```python
from build123d import *

# Parameters (mm, degrees)
BOSS_EXTRUDE1_DEPTH   = 46.39999966
SKETCH2_R             = 1.35
CUT_EXTRUDE1_DEPTH    = 57.705554564
CUT_EXTRUDE2_DEPTH    = 57.705554564
CUT_EXTRUDE3_DEPTH    = 77.912417193
MOVE_FACE1_BY         = 0.5
MOVE_FACE1_2_BY       = 0.5
CUT_EXTRUDE5_DEPTH    = 0.5
CUT_EXTRUDE6_DEPTH    = 0.5
MOVE_START            = 2.95
MOVE_FACE2_OUTLINE_W  = 4.2
MOVE_FACE2_OUTLINE_H  = 47.39999966
MOVE_FACE2_OUTLINE_R  = 1.35
MOVE_FACE2_DEPTH      = 2
MOVE_FACE3_BY         = 2
MOVE_FACE4_BY         = 0.1
MOVE_FACE4_2_BY       = 0.1
MOVE_FACE4_3_BY       = 0.1
MOVE_FACE4_4_BY       = 0.1
SKETCH14_W            = 31.645569848
SKETCH14_H            = 25
BOSS_EXTRUDE4_DEPTH   = 4
SKETCH15_R            = 2.1
CUT_EXTRUDE9_DEPTH    = 59.746648569
SKETCH16_R            = 3.6
CUT_EXTRUDE10_DEPTH   = 4.2
MOVE_FACE5_BY         = 4
MOVE_FACE6_BY         = 1
FILLET1_R             = 1
DELETEFACE1_START     = -5
DELETEFACE1_OUTLINE_R = 3.6
DELETEFACE1_DEPTH     = 6
DELETEFACE2_START     = -5
DELETEFACE2_OUTLINE_R = 1.35
DELETEFACE2_DEPTH     = 7.95
MOVE_FACE7_BY         = 4


# Read off the part's stored shape, not the designer's step: Move Face2, DeleteFace1, DeleteFace2
with BuildPart() as part:
    # Sketch1 → Boss-Extrude1 (new body)
    with BuildSketch(Plane.XY):
        Polygon((0, 0), (30, 0), (30, 12.7499), (22.3001, 12.7499), (22.3001, 9.7499), (26, 6.05), (26, 4.95), (22.3, 4.95), (22.3, 1), (0, 1), align=None)
    extrude(amount=-BOSS_EXTRUDE1_DEPTH)

    # Mirror1: part across plane


with BuildPart() as part_1:
    add(part.part)
    add(part.part.mirror(Plane(origin=(0, 1, -46.39999966), x_dir=(0, 0, 1), z_dir=(-1, 0, 0))))

    # Sketch2 → Cut-Extrude1 (cut, through all)
    with BuildSketch(Plane(origin=(0, 12.7499, 0), x_dir=(1, 0, 0), z_dir=(0, 1, 0))):
        with Locations(Location((-24.549999831, 1.999999999, 0), (0, 0, 270))):
            Circle(SKETCH2_R)
        with Locations(Location((-24.549999831, 44.399999661, 0), (0, 0, 270))):
            Circle(SKETCH2_R)
        with Locations(Location((24.549999831, 1.999999999, 0), (0, 0, 270))):
            Circle(SKETCH2_R)
        with Locations(Location((24.549999831, 44.399999661, 0), (0, 0, 270))):
            Circle(SKETCH2_R)
    extrude(amount=-CUT_EXTRUDE1_DEPTH, mode=Mode.SUBTRACT)

    # Sketch3 → Cut-Extrude2 (cut, through all)
    with BuildSketch(Plane.XY):
        Polygon((26.3, 12.7499), (30, 9.0499), (30, 12.7499), align=None)
        Polygon((-30, 12.7499), (-30, 9.0499), (-26.3, 12.7499), align=None)
    extrude(amount=-CUT_EXTRUDE2_DEPTH, mode=Mode.SUBTRACT)

    # Sketch4 → Cut-Extrude3 (cut, through all)
    with BuildSketch(Plane(origin=(30, 0, 0), x_dir=(0, 0, -1), z_dir=(1, 0, 0))):
        Polygon((9.19999983, 12.7499), (37.19999983, 12.7499), (30.416191902, 1), (15.983807758, 1), align=None)
    extrude(amount=-CUT_EXTRUDE3_DEPTH, mode=Mode.SUBTRACT)

    # Move Face1: a face moved outward by 0.5
    extrude(part_1.faces().sort_by_distance((-24, 3.187475, -46.39999966))[0], amount=MOVE_FACE1_BY, dir=(0, 0, -1))

    # Move Face1 2: a face moved outward by 0.5
    extrude(part_1.faces().sort_by_distance((-24, 3.187475, 0))[0], amount=MOVE_FACE1_2_BY, dir=(0, 0, 1))

    # Sketch6 → Cut-Extrude5 (cut)
    with BuildSketch(Plane(origin=(-26, 0, 0), x_dir=(0, 0, -1), z_dir=(1, 0, 0))):
        Polygon((13.703274195, 4.95), (13.068188899, 6.05), (-0.5, 6.05), (-0.5, 4.95), align=None)
        Polygon((33.331810761, 6.05), (32.696725465, 4.95), (46.89999966, 4.95), (46.89999966, 6.05), align=None)
    extrude(amount=-CUT_EXTRUDE5_DEPTH, mode=Mode.SUBTRACT)

    # Sketch7 → Cut-Extrude6 (cut)
    with BuildSketch(Plane.ZY.offset(-26)):
        Polygon((-13.068188899, 6.05), (-13.703274195, 4.95), (0.5, 4.95), (0.5, 6.05), align=None)
        Polygon((-32.696725465, 4.95), (-33.331810761, 6.05), (-46.89999966, 6.05), (-46.89999966, 4.95), align=None)
    extrude(amount=-CUT_EXTRUDE6_DEPTH, mode=Mode.SUBTRACT)

    # Move Face2 outline → Move Face2 (cut)
    # profile 1 of 2: a face of its own
    with BuildSketch(Plane(origin=(0, 0, 0), x_dir=(1, 0, 0), z_dir=(0, 1, 0)).offset(MOVE_START)):
        with Locations((-24.4, 23.19999983)):
            Rectangle(MOVE_FACE2_OUTLINE_W, MOVE_FACE2_OUTLINE_H)
        with Locations((-24.549999831, 1.999999999)):
            Circle(MOVE_FACE2_OUTLINE_R, mode=Mode.SUBTRACT)
        with Locations((-24.549999831, 44.399999661)):
            Circle(MOVE_FACE2_OUTLINE_R, mode=Mode.SUBTRACT)
    # profile 2 of 2: a face of its own
    with BuildSketch(Plane(origin=(0, 0, 0), x_dir=(1, 0, 0), z_dir=(0, 1, 0)).offset(MOVE_START)):
        with Locations((24.4, 23.19999983)):
            Rectangle(MOVE_FACE2_OUTLINE_W, MOVE_FACE2_OUTLINE_H)
        with Locations((24.549999831, 1.999999999)):
            Circle(MOVE_FACE2_OUTLINE_R, mode=Mode.SUBTRACT)
        with Locations((24.549999831, 44.399999661)):
            Circle(MOVE_FACE2_OUTLINE_R, mode=Mode.SUBTRACT)
    extrude(amount=MOVE_FACE2_DEPTH, mode=Mode.SUBTRACT)

    # Move Face3: a face moved outward by 2.0
    extrude(part_1.faces().sort_by_distance((0, 0, -23.19999983))[0], amount=MOVE_FACE3_BY, dir=(0, -1, 0))

    # Move Face4: a face moved inward by 0.1
    extrude(part_1.faces().sort_by_distance((-26.5, 4.468031617, -6.740769385))[0], amount=MOVE_FACE4_BY, dir=(-1, 0, 0), mode=Mode.SUBTRACT)

    # Move Face4 2: a face moved inward by 0.1
    extrude(part_1.faces().sort_by_distance((-26.5, 4.468031617, -39.659230275))[0], amount=MOVE_FACE4_2_BY, dir=(-1, 0, 0), mode=Mode.SUBTRACT)

    # Move Face4 3: a face moved inward by 0.1
    extrude(part_1.faces().sort_by_distance((26.5, 4.468031617, -6.740769385))[0], amount=MOVE_FACE4_3_BY, dir=(1, 0, 0), mode=Mode.SUBTRACT)

    # Move Face4 4: a face moved inward by 0.1
    extrude(part_1.faces().sort_by_distance((26.5, 4.468031617, -39.659230275))[0], amount=MOVE_FACE4_4_BY, dir=(1, 0, 0), mode=Mode.SUBTRACT)

    # Sketch14 → Boss-Extrude4 (add)
    with BuildSketch(Plane.XZ.offset(2)):
        with Locations((0, -23.19999983)):
            Rectangle(SKETCH14_W, SKETCH14_H)
    extrude(amount=BOSS_EXTRUDE4_DEPTH)

    # Sketch15 → Cut-Extrude9 (cut, through all)
    with BuildSketch(Plane.XZ.offset(6)):
        with Locations(Location((-8.5, -14.69999983, 0), (0, 0, 270))):
            Circle(SKETCH15_R)
        with Locations(Location((8.5, -14.69999983, 0), (0, 0, 270))):
            Circle(SKETCH15_R)
        with Locations(Location((8.5, -31.69999983, 0), (0, 0, 270))):
            Circle(SKETCH15_R)
        with Locations(Location((-8.5, -31.69999983, 0), (0, 0, 270))):
            Circle(SKETCH15_R)
    extrude(amount=-CUT_EXTRUDE9_DEPTH, mode=Mode.SUBTRACT)

    # Sketch16 → Cut-Extrude10 (cut)
    with BuildSketch(Plane(origin=(0, 1, 0), x_dir=(1, 0, 0), z_dir=(0, 1, 0))):
        with Locations(Location((-8.5, 31.69999983, 0), (0, 0, 270))):
            Circle(SKETCH16_R)
        with Locations(Location((8.5, 31.69999983, 0), (0, 0, 270))):
            Circle(SKETCH16_R)
        with Locations(Location((8.5, 14.69999983, 0), (0, 0, 270))):
            Circle(SKETCH16_R)
        with Locations(Location((-8.5, 14.69999983, 0), (0, 0, 270))):
            Circle(SKETCH16_R)
    extrude(amount=-CUT_EXTRUDE10_DEPTH, mode=Mode.SUBTRACT)

    # Move Face5: a face moved outward by 4.0
    extrude(part_1.faces().sort_by_distance((0, -2, -42.159999694))[0], amount=MOVE_FACE5_BY, dir=(0, -1, 0))

    # Move Face6: a face moved inward by 1.0
    extrude(part_1.faces().sort_by_distance((0, -6, -23.19999983))[0], amount=MOVE_FACE6_BY, dir=(0, 1, 0), mode=Mode.SUBTRACT)

    # Fillet1
    fillet1_edges = [part_1.edges().sort_by_distance(p)[0] for p in [
        (30, 2.02495, -46.89999966),
        (30, 2.02495, 0.5),
        (-30, 2.02495, 0.5),
        (-30, 2.02495, -46.89999966),
        (28.15, 10.8999, -46.89999966),
        (28.15, 10.8999, 0.5),
        (-28.15, 10.8999, -46.89999966),
        (-28.15, 10.8999, 0.5),
    ]]
    fillet(fillet1_edges, radius=FILLET1_R)

    # DeleteFace1 outline → DeleteFace1 (add)
    with BuildSketch(Plane(origin=(0, 0, 0), x_dir=(1, 0, 0), z_dir=(0, 1, 0)).offset(DELETEFACE1_START)):
        with Locations((-8.5, 14.69999983)):
            Circle(DELETEFACE1_OUTLINE_R)
        with Locations((8.5, 14.69999983)):
            Circle(DELETEFACE1_OUTLINE_R)
        with Locations((8.5, 31.69999983)):
            Circle(DELETEFACE1_OUTLINE_R)
        with Locations((-8.5, 31.69999983)):
            Circle(DELETEFACE1_OUTLINE_R)
    extrude(amount=DELETEFACE1_DEPTH)

    # DeleteFace2 outline → DeleteFace2 (add)
    with BuildSketch(Plane(origin=(0, 0, 0), x_dir=(1, 0, 0), z_dir=(0, 1, 0)).offset(DELETEFACE2_START)):
        with Locations((-24.549999831, 1.999999999)):
            Circle(DELETEFACE2_OUTLINE_R)
        with Locations((-24.549999831, 44.399999661)):
            Circle(DELETEFACE2_OUTLINE_R)
        with Locations((24.549999831, 1.999999999)):
            Circle(DELETEFACE2_OUTLINE_R)
        with Locations((24.549999831, 44.399999661)):
            Circle(DELETEFACE2_OUTLINE_R)
    extrude(amount=DELETEFACE2_DEPTH)

    # Move Face7: a face moved inward by 4.0
    extrude(part_1.faces().sort_by_distance((0, -5, -23.19999983))[0], amount=MOVE_FACE7_BY, dir=(0, 1, 0), mode=Mode.SUBTRACT)


solid = part_1.part
```
Part model, mm, in its own coordinate system. A direction names the side the tool comes from. Round coordinates to 2 decimals unless told otherwise and drop trailing zeros. Order: outer loops, then holes, each group sorted by start corner. A loop starts at its lowest first (then second) coordinate and runs counter-clockwise, first axis right, second up. Notation, with made-up numbers: M 55,58 L 82,58 A16 ccw 82,77 Z; hole C 25,6 d4. An arc over 180 degrees is marked long. Put each result on its own line as item: value. Start each with the question number.
1. Slice it at C-C on x = -3. List the corners of the cut face in (y, z), then the cut area to 3 significant figures.
2. Tool access for faces 1 (the face through (-26.1, 6.79, -12.64)), 2 (the face through (25.889, 10.217, -44.576)), 3 (the face through (-24, 2.95, -7)), 4 (the face through (-22.3, 2, -8)): list every direction of +Z, -Z, +X, -X, +Y, -Y with a clear straight run to the whole face (end or side of a thin tool).
3. Slice it at D-D on z = -23. List the corners of the cut face in (x, y).
4. Drop flat-ended pins along their axis: pin 1 (3 mm diameter, centred on x = 22.5, z = -33, fed in from +Y); pin 2 (12 mm diameter, centred on x = 3.5, z = -22, fed in from +Y); pin 3 (1.6 mm diameter, centred on x = 24.55, z = -44.4, fed in from +Y). Give the stop position or say it passes through.
5. Two-plate mould, pull along Y, no slides. Class faces 5 (the face through (24, 12.75, -4)), 6 (the face through (25.889, 10.217, -2.176)), 7 (the face through (24, 2.95, -7)), 8 (the face through (0, -1, -24)): +Y half, -Y half, draft (parallel to the pull), parting line (faces both ways), or undercut.
6. Slice it at A-A on z = -2. List the corners of the cut face in (x, y), then the cut area to 3 significant figures.
7. Drill centre lines: probe 1 along X at (y, z) = (8, -44.4); probe 2 along Z at (x, y) = (24.55, 10.5); probe 3 along X at (y, z) = (2.25, -42.5). Where is each one in solid material? Low to high. Write a range as [from, to].
8. Slice it at B-B on z = -36.5. List the corners of the cut face in (x, y).
Findings:
1. outline: M -1,-46.9 L 1,-46.9 L 1,0.5 L -1,0.5 Z
1. area: 94.8 mm2
2. face 1: +X, -X, +Y
2. face 2: +Y
2. face 3: +Z, -Z
2. face 4: +Z, -Z, +Y
3. outline: M -30,-1 L 30,-1 L 30,1 L -30,1 Z
4. pin 1: y = 2.95
4. pin 2: y = 1
4. pin 3: y = 2.95
5. face 5: +Y half
5. face 6: draft
5. face 7: undercut
5. face 8: -Y half
6. outline: M -30,-1 L 30,-1 L 30,9.05 L 26.3,12.75 L 25.9,12.75 L 25.9,6.15 L 26,6.05 L 26.6,6.05 L 26.6,2.95 L 22.3,2.95 L 22.3,1 L -22.3,1 L -22.3,2.95 L -26.6,2.95 L -26.6,6.05 L -26,6.05 L -25.9,6.15 L -25.9,12.75 L -26.3,12.75 L -30,9.05 Z; M -23.2,8.85 L -22.3,9.75 L -22.3,12.75 L -23.2,12.75 Z; M 22.3,9.75 L 23.2,8.85 L 23.2,12.75 L 22.3,12.75 Z
6. area: 219 mm2
7. probe 1: [-30, -25.9], [25.9, 30]
7. probe 2: [-46.9, -45.75], [-43.05, -35.9], [-10.5, -3.35], [-0.65, 0.5]
7. probe 3: [-30, -22.3], [22.3, 30]
8. outline: M -30,-1 L 30,-1 L 30,9.05 L 27.51,11.54 L 22.3,11.54 L 22.3,9.75 L 26,6.05 L 26.6,6.05 L 26.6,2.95 L 22.3,2.95 L 22.3,1 L -22.3,1 L -22.3,2.95 L -26.6,2.95 L -26.6,6.05 L -26,6.05 L -22.3,9.75 L -22.3,11.54 L -27.51,11.54 L -30,9.05 Z
